Verification items for the finished model (mm, model axes). Face numbers are marked on the shaded views. Round coordinates to 2 decimals unless told otherwise and drop trailing zeros. Order: outer loops, then holes, each group sorted by start corner. A loop starts at its lowest first (then second) coordinate and runs counter-clockwise, first axis right, second up. Notation, with made-up numbers: M 85,13 L 139,13 A24 ccw 139,30 Z; hole C 51,43 d8. An arc over 180 degrees is marked long. Use CSV: the item, a comma, the result in double quotes. Start each with the question number.
Q1. Mould release check, pull along Y, two halves, no side actions. Record for the marked faces 1, 2, 3 and 4: +Y half, -Y half, draft (parallel to the pull), parting line (faces both ways), or undercut.
Q2. Sectioned sample at C-C (z = -2). Enter the section's corners in (x, y), and give its area (3 significant figures).
Q3. Sectioned sample at B-B (x = 0.75). Enter the section's corners in (y, z), and give its area (3 significant figures).
Q4. Scan lines: line 1 (Y direction, x = 1.95, z = -2); line 2 (Z direction, x = 2.25, y = 9.5); line 3 (Y direction, x = 0.3, z = -2.75). Record each from-to range of solid material in increasing order.
Q5. Gauge pin test, flat ends, axial feed: pin 1 Ø3 at (y, z) = (3, 3.5) entering from -X; pin 2 Ø0.8 at (x, z) = (3, 2.5) entering from +Y; pin 3 Ø4 at (y, z) = (-11.5, -2) entering from +X; pin 4 Ø1.6 at (x, z) = (3.5, 1.5) entering from -Y. Record the tip position at first contact, or that the pin passes through.
Q6. Sectioned sample at A-A (y = -11.5). Enter the section's corners in (x, z), and give its area (3 significant figures).
Q7. Sectioned sample at D-D (y = 1). Enter the section's corners in (x, z).
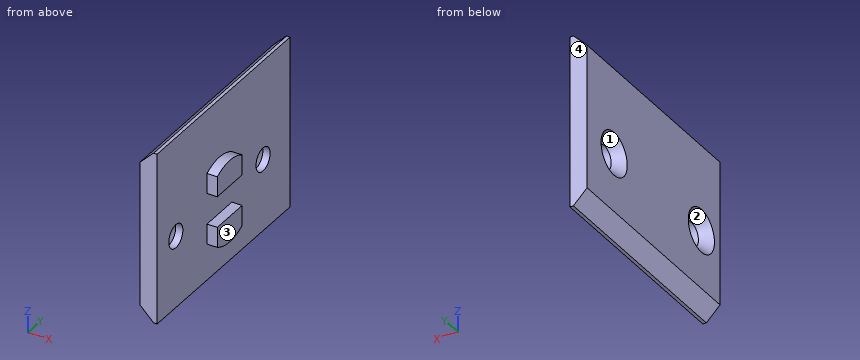
```python
from build123d import *

# Parameters (mm, degrees)
SKETCH_1_W                 = 25
SKETCH_1_H                 = 32
EXTRUDE_1_DEPTH            = 2.5
CHAMFER_1_SIZE             = 2
HOLE_WIZARD_M31_AT_2_COUNT = 2
HOLE_WIZARD_M31_AT_2_PITCH = 21
SKETCH_4_R                 = 6
SKETCH_4_R_2               = 3.5
EXTRUDE_2_DEPTH            = 1.5
SKETCH_5_W                 = 4.5
SKETCH_5_H                 = 16
CUT_EXTRUDE_1_DEPTH        = 1.5
CUT_EXTRUDE_2_DEPTH        = 1.5


with BuildPart() as part:
    # Эскиз1 → Бобышка-Вытянуть1 (new body)
    with BuildSketch(Plane(origin=(0, 0, 0), x_dir=(0, 0, -1), z_dir=(1, 0, 0))):
        Rectangle(SKETCH_1_W, SKETCH_1_H)
    extrude(amount=EXTRUDE_1_DEPTH)

    # Фаска1
    chamfer_1_edges = [part.edges().sort_by_distance(p)[0] for p in [
        (0, 0, 12.5),
        (0, 0, -12.5),
    ]]
    chamfer(chamfer_1_edges, length=CHAMFER_1_SIZE)

    # Эскиз3 → Зенковка для  винта с плоской головкой M31 (revolve, cut)
    with BuildSketch(Plane(origin=(0, -11.5, -2), x_dir=(0, 0, 1), z_dir=(0, 1, 0))):
        Polygon((0, 0), (0, 2.5), (1.7, 2.5), (1.7, 1.45), (3.15, 0), align=None)
    hole_wizard_m31 = revolve(axis=Axis((-6.35, -11.5, -2), (1, 0, 0)), mode=Mode.SUBTRACT)

    # Зенковка для  винта с плоской головкой M31 at 2: Зенковка для  винта с плоской головкой M31 ×2
    with Locations(*[(0, i * HOLE_WIZARD_M31_AT_2_PITCH, 0) for i in range(1, HOLE_WIZARD_M31_AT_2_COUNT)]):
        add(hole_wizard_m31, mode=Mode.SUBTRACT)

    # Эскиз4 → Бобышка-Вытянуть2 (add)
    with BuildSketch(Plane(origin=(2.5, 0, 0), x_dir=(0, 0, -1), z_dir=(1, 0, 0))):
        with Locations((2, -1)):
            Circle(SKETCH_4_R)
        with Locations((2, -1)):
            Circle(SKETCH_4_R_2, mode=Mode.SUBTRACT)
        with BuildLine():
            ThreePointArc((-0.25, 1.680951324), (-1.5, -1), (-0.25, -3.680951324))
            Line((-0.25, -3.680951324), (-0.25, 1.680951324))
        make_face()
        with BuildLine():
            Line((4.25, 1.680951324), (4.25, -3.680951324))
            ThreePointArc((4.25, -3.680951324), (5.172144385, -2.479019946), (5.5, -1))
            ThreePointArc((5.5, -1), (5.172144385, 0.479019946), (4.25, 1.680951324))
        make_face()
    extrude(amount=EXTRUDE_2_DEPTH)

    # Эскиз5 → Вырез-Вытянуть1 (cut)
    with BuildSketch(Plane(origin=(4, 0, 0), x_dir=(0, 0, -1), z_dir=(1, 0, 0))):
        with Locations((2, -1)):
            Rectangle(SKETCH_5_W, SKETCH_5_H)
    extrude(amount=-CUT_EXTRUDE_1_DEPTH, mode=Mode.SUBTRACT)

    # Эскиз6 → Вырез-Вытянуть2 (cut)
    with BuildSketch(Plane(origin=(4, 0, 0), x_dir=(0, 0, -1), z_dir=(1, 0, 0))):
        with BuildLine():
            ThreePointArc((4.25, 4.562148865), (0.047794779, 4.67352578), (-3.196152423, 2))
            Line((-3.196152423, 2), (4.25, 2))
            Line((4.25, 2), (4.25, 4.562148865))
        make_face()
        with BuildLine():
            Line((4.25, 4.562148865), (4.25, 2))
            Line((4.25, 2), (7.196152423, 2))
            ThreePointArc((7.196152423, 2), (5.937314844, 3.527422205), (4.25, 4.562148865))
        make_face()
        with BuildLine():
            Line((4.25, -4), (-3.196152423, -4))
            ThreePointArc((-3.196152423, -4), (0.047794779, -6.67352578), (4.25, -6.562148865))
            Line((4.25, -6.562148865), (4.25, -4))
        make_face()
        with BuildLine():
            Line((7.196152423, -4), (4.25, -4))
            Line((4.25, -4), (4.25, -6.562148865))
            ThreePointArc((4.25, -6.562148865), (5.937314844, -5.527422205), (7.196152423, -4))
        make_face()
    extrude(amount=-CUT_EXTRUDE_2_DEPTH, mode=Mode.SUBTRACT)


solid = part.part
```
Verdict:
1,face 1,"undercut"
1,face 2,"undercut"
1,face 3,"draft"
1,face 4,"+Y half"
2,outline,"M 0,-16 L 2.5,-16 L 2.5,-13.2 L 1.45,-13.2 L 0,-14.65 Z; M 0,-8.35 L 1.45,-9.8 L 2.5,-9.8 L 2.5,7.8 L 1.45,7.8 L 0,6.35 Z; M 0,12.65 L 1.45,11.2 L 2.5,11.2 L 2.5,16 L 0,16 Z"
2,area,"58.8 mm²"
3,outline,"M -16,-11.25 L 16,-11.25 L 16,11.25 L -16,11.25 Z; hole C -11.5,-2 d4.8; hole C 9.5,-2 d4.8"
3,area,"684 mm²"
4,line 1,"y = -16 to -13.2, -9.8 to 7.8, 11.2 to 16"
4,line 2,"z = -12.5 to -3.7, -0.3 to 12.5"
4,line 3,"y = -16 to -14.25, -8.75 to 6.75, 12.25 to 16"
5,pin 1,"stops at x = 0"
5,pin 2,"stops at y = 2"
5,pin 3,"stops at x = 2.5"
5,pin 4,"stops at y = -4"
6,outline,"M 0,-10.5 L 2,-12.5 L 2.5,-12.5 L 2.5,-3.7 L 1.45,-3.7 L 0,-5.15 Z; M 0,1.15 L 1.45,-0.3 L 2.5,-0.3 L 2.5,12.5 L 2,12.5 L 0,10.5 Z"
6,area,"47.9 mm²"
7,outline,"M 0,-10.5 L 2,-12.5 L 2.5,-12.5 L 2.5,-7.66 L 4,-7.66 L 4,-4.25 L 2.5,-4.25 L 2.5,0.25 L 4,0.25 L 4,3.66 L 2.5,3.66 L 2.5,12.5 L 2,12.5 L 0,10.5 Z"
